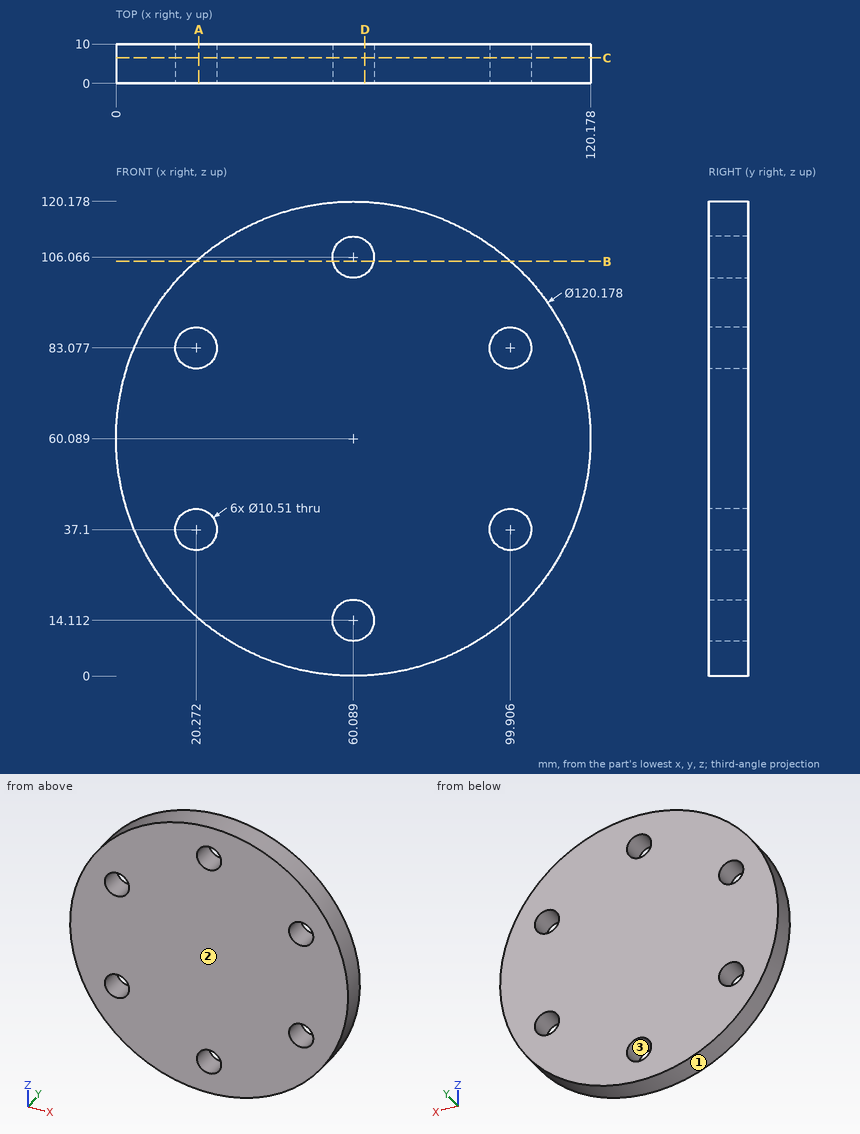
Source: three-view drawing plus pictorial views. Frame: mm from the lowest corner of the part. Coordinates: 2 decimals unless noted, no trailing zeros. Write each loop counter-clockwise with the first axis right and the second up, starting at its lowest first coordinate (ties: lowest second). Pieces come first, ordered by that corner, then holes. Notation, with made-up numbers: (-35, 65.25) - (4, 65.25) arc R23 cw to (4, 102.25) - close; hole circle Ø10 at (18.25, 20.5). An arc over 180 degrees is marked (long way). Return JSON: item names as keys, results as strings.
Item 1: Section query B-B (z = 105). Output: boundary loops of the cut face in (x, y) (1 decimal).
Completed:
{"outline": "(20.2, 0) - (54.9, 0) - (54.9, 10) - (20.2, 10) - close; (65.2, 0) - (100, 0) - (100, 10) - (65.2, 10) - close"}
Item 2: Section query D-D (x = 63). Output: boundary loops of the cut face in (y, z), and give its area (3 significant figures).
Completed:
{"outline": "(0, 0.07) - (10, 0.07) - (10, 9.74) - (0, 9.74) - close; (0, 18.49) - (10, 18.49) - (10, 101.69) - (0, 101.69) - close; (0, 110.44) - (10, 110.44) - (10, 120.11) - (0, 120.11) - close", "area": "1,030 mm2"}
Item 3: Pin query (flat end, axial travel): pin 1 Ø1.5 at (y, z) = (5.5, 102.5) entering from -X; pin 2 Ø1 at (y, z) = (8, 88) entering from +X; pin 3 Ø9.5 at (x, z) = (99.91, 37.1) entering from +Y; pin 4 Ø17 at (x, z) = (20.27, 37.1) entering from -Y. Return the tip coordinate at first contact, or that it passes through.
Completed:
{"pin 1": "stops at x = 16.79", "pin 2": "stops at x = 113.56", "pin 3": "passes through", "pin 4": "stops at y = 0"}
Item 4: Line query: L1, parallel to Z at x = 60, y = 6; L2, parallel to X at y = 5.75, z = 37 (1 decimal); L3, parallel to X at y = 7, z = 84.5 (1 decimal). Output: solid intervals per line, ascending.
Completed:
{"L1": "z = 0 to 8.86, 19.37 to 100.81, 111.32 to 120.18", "L2": "x = 4.6 to 15, 25.5 to 94.7, 105.2 to 115.6", "L3": "x = 5.2 to 15.2, 25.3 to 94.8, 105 to 115"}
Item 5: Section query A-A (x = 21). Output: boundary loops of the cut face in (y, z) (1 decimal).
Completed:
{"outline": "(0, 14.5) - (10, 14.5) - (10, 31.9) - (0, 31.9) - close; (0, 42.3) - (10, 42.3) - (10, 77.9) - (0, 77.9) - close; (0, 88.3) - (10, 88.3) - (10, 105.7) - (0, 105.7) - close"}
Item 6: Pull-direction query (Z, two-part tool) for the marked faces 1, 2 and 3; classes: +Z half, -Z half, draft (parallel to the pull), parting line (faces both ways), or undercut.
Completed:
{"face 1": "parting line", "face 2": "draft", "face 3": "undercut"}
Item 7: Section query C-C (y = 6.5). Count the separate pieces of the cut face and the enclosed holes in it, and give its area (3 significant figures).
Completed:
{"separate pieces": "1", "enclosed holes": "6", "area": "10,800 mm2"}
